from build123d import *

# Parameters (mm, degrees)
F0_W     = 300
F0_H     = 100
F1_DEPTH = 9
F3_DEPTH = 300.001
F4_R     = 1.49999
F5_R     = 5.99999


# Not quite as in the source:
# - a fillet or chamfer is up to 0.001 mm smaller than in the source, because OpenCascade refuses the exact size


with BuildPart() as f1:
    # F0 (on Front) → F1 (new body, symmetric)
    with BuildSketch(Plane.XZ):
        with Locations((-3.7248600274, -105.7776198197)):
            Rectangle(F0_W, F0_H)
    extrude(amount=F1_DEPTH, both=True)

    # F2 (on face) → F3 (cut, through all)
    with BuildSketch(Plane.YZ.offset(146.2751399726)):
        Polygon((6, -55.7776198197), (-9, -55.7776198197), (-9, -72.7776198197), (-6, -72.7776198197), (-6, -80.7776198197), (6, -80.7776198197), align=None)
    extrude(amount=-F3_DEPTH, mode=Mode.SUBTRACT)

    # F4 (radius 1.5 in the source; OpenCascade refuses exactly that, so slightly less here)
    f4_edges = [f1.edges().sort_by_distance(p)[0] for p in [
        (-3.72486, 6, -55.77762),
        (-3.72486, 9, -55.77762),
        (-3.72486, -9, -72.77762),
        (-3.72486, -6, -72.77762),
    ]]
    fillet(f4_edges, radius=F4_R)

    # F5 (radius 6 in the source; OpenCascade refuses exactly that, so slightly less here)
    f5_edges = [f1.edges().sort_by_distance(p)[0] for p in [
        (-3.72486, 6, -80.77762),
        (-3.72486, -6, -80.77762),
    ]]
    fillet(f5_edges, radius=F5_R)


solid = f1.part
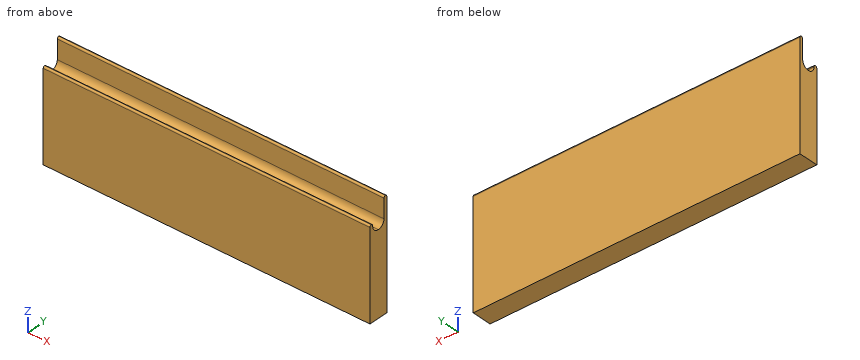
The model under review builds one solid part; all positions refer to its coordinate system, in mm. Round coordinates to 2 decimals unless told otherwise and drop trailing zeros. Write each loop counter-clockwise with the first axis right and the second up, starting at its lowest first coordinate (ties: lowest second). Pieces come first, ordered by that corner, then holes. Notation, with made-up numbers: (11, 17.5) -> (53, 17.5) arc R20 ccw to (53, 26.5) -> close; hole circle Ø8 at (48, 84). An arc over 180 degrees is marked (long way). Answer as a JSON object with one key per item and string values.
1. Clearance check with flat-ended pins moving along their axes: pin 1 (5 mm diameter, centred on x = -17, y = 6, fed in from +Z); pin 2 (9 mm diameter, centred on x = -16.5, z = -67.5, fed in from -Y); pin 3 (6 mm diameter, centred on x = -1.5, y = -6, fed in from +Z); pin 4 (3 mm diameter, centred on x = 80, y = -3.5, fed in from +Z). State where each tip first meets the part, or that it passes through.
Results found:
{"pin 1": "stops at z = -55.78", "pin 2": "stops at y = 6", "pin 3": "stops at z = -72.78", "pin 4": "stops at z = -78.09"}
2. We need section B-B on y = -2.75. State the section outline as (x, z) points.
Results found:
{"outline": "(-153.72, -155.78) -> (146.28, -155.78) -> (146.28, -80.11) -> (-153.72, -80.11) -> close"}
3. To check wall thickness, follow line 1 along Y through (x, z) = (-95, -60.5); line 2 along Z through (x, y) = (-3.5, -0.75); line 3 along Z through (x, y) = (-5, -4.75). State the ranges of each line that lie inside material, in increasing order.
Results found:
{"line 1": "y = 6 to 9", "line 2": "z = -155.78 to -80.73", "line 3": "z = -155.78 to -78.44"}
